Part model, mm, in its own coordinate system. Face numbers are marked on the shaded views. A direction names the side the tool comes from. Round coordinates to 2 decimals unless told otherwise and drop trailing zeros. Loops run counter-clockwise (first coordinate to the right, second up) from the corner with the lowest first, then second, coordinate; pieces in that order, holes last. Notation, with made-up numbers: M 68.25,5.5 L 111.25,5.5 A15 ccw 111.25,26.5 Z; hole C 85.5,18.25 d11. An arc over 180 degrees is marked long. Put each result on its own line as item: value. Start each with the question number.
```python
from build123d import *

# Parameters (mm, degrees)
SKETCH1_R           = 50
BOSS_EXTRUDE1_DEPTH = 400
SKETCH3_R           = 10
BOSS_EXTRUDE2_DEPTH = 10
SHELL1_START        = 30
SHELL1_OUTLINE_R    = 20
SHELL1_DEPTH        = 370


# Read off the part's stored shape, not the designer's step: Shell1
with BuildPart() as part:
    # Sketch1 → Boss-Extrude1 (new body)
    with BuildSketch(Plane.XY):
        Circle(SKETCH1_R)
    extrude(amount=BOSS_EXTRUDE1_DEPTH)

    # Sketch3 → Boss-Extrude2 (add, symmetric)
    with BuildSketch(Plane(origin=(0, 0, 0), x_dir=(1, 0, 0), z_dir=(0, 1, 0))):
        with BuildLine():
            ThreePointArc((-30, 45), (0, 75), (30, 45))
            Line((30, 45), (45, 0))
            Line((45, 0), (-45, 0))
            Line((-45, 0), (-30, 45))
        make_face()
        with Locations(Location((0, 45, 0), (0, 0, 270))):
            Circle(SKETCH3_R, mode=Mode.SUBTRACT)
    extrude(amount=BOSS_EXTRUDE2_DEPTH, both=True)

    # Shell1 outline → Shell1 (cut)
    with BuildSketch(Plane.XY.offset(SHELL1_START)):
        Circle(SHELL1_OUTLINE_R)
    extrude(amount=SHELL1_DEPTH, mode=Mode.SUBTRACT)


solid = part.part
```
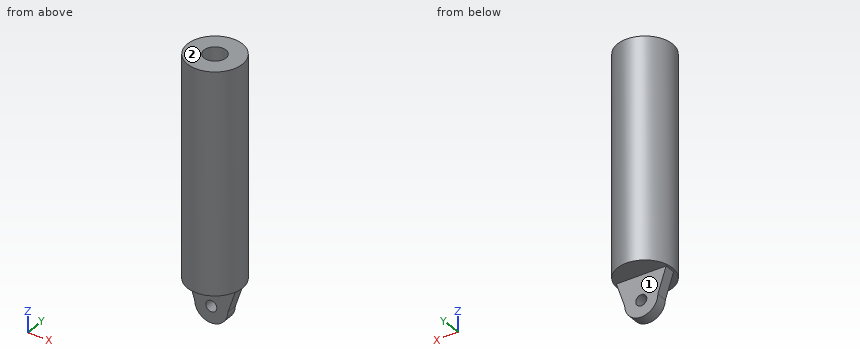
1. Wall check: L1, parallel to X at y = -5.75, z = -45; L2, parallel to X at y = -1, z = 170.5; L3, parallel to Y at x = 0, z = 259.5. Give the ranges that are in metal, low to high.
2. Cut at C-C, the plane z = 45.5. Give the cut face in (x, y), and give its area (3 significant figures).
3. Which spindle directions (+Z, -Z, +X, -X, +Y, -Y) get a long thin tool onto all of the face, cutting with end or side? Do the marked faces 1 and 2. Say none if no direction does.
4. Cut at D-D, the plane y = -40. Give the cut face in (x, z), and give its area (3 significant figures).
5. Cut at B-B, the plane y = 0. Give the cut face in (x, z).
6. Cut at A-A, the plane x = 0. Give the cut face in (y, z), and give its area (3 significant figures).
7. Drop flat-ended pins along their axis: pin 1 (10 mm diameter, centred on x = 8, z = 200.5, fed in from +Y); pin 2 (3 mm diameter, centred on x = 15, z = 46.5, fed in from +Y); pin 3 (10 mm diameter, centred on x = 4.5, z = 239, fed in from -Y); pin 4 (18 mm diameter, centred on x = 0, z = -45, fed in from +Y). Give the stop position or say it passes through.
Results list:
1. L1: x = -30 to -10, 10 to 30
1. L2: x = -49.99 to -19.97, 19.97 to 49.99
1. L3: y = -50 to -20, 20 to 50
2. outline: C 0,0 d100; hole C 0,0 d40
2. area: 6,600 mm^2
3. face 1: -Z, +X, -X, +Y
3. face 2: +Z, +X, -X, +Y, -Y
4. outline: M -30,0 L 30,0 L 30,400 L -30,400 Z
4. area: 24,000 mm^2
5. outline: M -50,0 L -45,0 L -30,-45 A30 ccw 30,-45 L 45,0 L 50,0 L 50,400 L 20,400 L 20,30 L -20,30 L -20,400 L -50,400 Z; hole C 0,-45 d20
6. outline: M -50,0 L -10,0 L -10,-35 L 10,-35 L 10,0 L 50,0 L 50,400 L 20,400 L 20,30 L -20,30 L -20,400 L -50,400 Z; M -10,-75 L 10,-75 L 10,-55 L -10,-55 Z
6. area: 26,300 mm^2
7. pin 1: stops at y = 49.91
7. pin 2: stops at y = 48.14
7. pin 3: stops at y = -50
7. pin 4: passes through
